Here's how the part is built. I have some questions about the finished solid (model axes, mm). A direction names the side the tool comes from. Round coordinates to 2 decimals unless told otherwise and drop trailing zeros. Order: outer loops, then holes, each group sorted by start corner. A loop starts at its lowest first (then second) coordinate and runs counter-clockwise, first axis right, second up. Notation, with made-up numbers: (84.25, 46) -> (100.25, 46) arc R21 ccw to (100.25, 67) -> close; hole circle Ø11 at (48.5, 7.5). An arc over 180 degrees is marked (long way). One line per item, written item: value.
```python
from build123d import *

# Parameters (mm, degrees)
F3_R     = 18
F4_DEPTH = 230


with BuildPart() as f1:
    # F0 (on Front) → F1 (revolve)
    with BuildSketch(Plane.XZ):
        Polygon((0, 234), (0, 0), (22, 0), (22, 201.5), (18.4, 201.5), (18.4, 204), (19.5, 204), (19.5, 234), align=None)
    revolve(axis=Axis((0, 0, 117), (0, 0, -1)))

    # F3 (on face) → F4 (cut)
    with BuildSketch(Plane.XY.offset(234)):
        Circle(F3_R)
    extrude(amount=-F4_DEPTH, mode=Mode.SUBTRACT)


solid = f1.part
```
Q1. For P1, Ø2, axis at y = 17.5, z = 101, coming from the +X side; P2, Ø8, axis at y = -16, z = 200.5, coming from the -X side; P3, Ø5, axis at x = 8.5, z = 53.5, coming from the -Y side, each with a flat end and sliding along its axis, tell me the tip position at first contact or that it passes through.
Answers:
P1: x = 14.55
P2: x = -18.44
P3: y = -21.17
Q2. Which directions (+Z, -Z, +X, -X, +Y, -Y) give clear straight access to the entire face, cutting with the end or side of a thin tool? Please do faces 5 (the face through (0, 0, 0)), 6 (the face through (-2.539, -19.334, 219.21)), 7 (the face through (-17.2, 7.1, 204)).
Answers:
face 5: -Z, +X, -X, +Y, -Y
face 6: +Z
face 7: none
Q3. I want a section at B-B on y = 0. Write out the boundary of the cut face in (x, z), then the cut area to 3 significant figures.
Answers:
outline: (-22, 0) -> (22, 0) -> (22, 201.5) -> (18.4, 201.5) -> (18.4, 204) -> (19.5, 204) -> (19.5, 234) -> (18, 234) -> (18, 4) -> (-18, 4) -> (-18, 234) -> (-19.5, 234) -> (-19.5, 204) -> (-18.4, 204) -> (-18.4, 201.5) -> (-22, 201.5) -> close
area: 1,850 mm2
Q4. If we mould it in two halves opening along Y, with no side actions, what happens to faces 1 (the face through (0, 0, 4)), 2 (the face through (-2.343, 17.847, 120.61)), 3 (the face through (5.69, 17.24, 234)), 4 (the face through (-4.769, 21.477, 102.16))? For each: pulls with the +Y half, pulls with the -Y half, needs draft (parallel to the pull), parting line crosses it, or undercut.
Answers:
face 1: undercut
face 2: undercut
face 3: needs draft
face 4: parting line crosses it
Q5. I want a section at A-A on z = 122. Write out the boundary of the cut face in (x, y).
Answers:
outline: circle Ø44 at (0, 0); hole circle Ø36 at (0, 0)
Q6. I need wall thicknesses on line 1 along Y through (x, z) = (0, 172); line 2 along Z through (x, y) = (0, 9.5); line 3 along X through (y, z) = (3.5, 107.5). Which ranges of each line are inside material? Lowest first, please.
Answers:
line 1: -22 to -18, 18 to 22
line 2: 0 to 4
line 3: -21.72 to -17.66, 17.66 to 21.72
